Model file for the job. Use its own axes, mm. A direction names the side the tool comes from. Coordinates: 2 decimals unless noted, no trailing zeros. Order: outer loops, then holes, each group sorted by start corner. A loop starts at its lowest first (then second) coordinate and runs counter-clockwise, first axis right, second up. Notation, with made-up numbers: M -4,17 L 48,17 A32 cw 48,51 Z; hole C 11,44.5 d5. An arc over 180 degrees is marked long. Return JSON: item names as keys, results as strings.
```python
from build123d import *
from build123d.topology import SkipClean

# Parameters (mm, degrees)
SKETCH_1_R           = 19.5
SKETCH_1_R_2         = 18
EXTRUDE_1_DEPTH      = 20
SKETCH_3_R           = 27.5
EXTRUDE_2_DEPTH      = 3
EXTRUDE_START        = 2
SKETCH_25_R          = 21.75
SKETCH_25_R_2        = 19.5
EXTRUDE_12_DEPTH     = 2
EXTRUDE_START_2      = -1
SKETCH_26_R          = 21.75
SKETCH_26_R_2        = 19.5
EXTRUDE_13_DEPTH     = 2
EXTRUDE_START_3      = -3
EXTRUDE_14_DEPTH     = 3
SKETCH_28_W          = 21.458236434
SKETCH_28_H          = 3
SKETCH_28_W_2        = 3.541763566
EXTRUDE_17_DEPTH     = 1.5
EXTRUDE_START_4      = -53.5
EXTRUDE_25_DEPTH     = 53.5
CUT_EXTRUDE_START    = -52
CUT_EXTRUDE_15_DEPTH = 52
EXTRUDE_24_DEPTH     = 11
CUT_EXTRUDE_START_2  = -1.5
CUT_EXTRUDE_10_DEPTH = 1.5
SKETCH_34_W          = 10.2
SKETCH_34_H          = 6.5
SKETCH_34_W_2        = 8.2
SKETCH_34_H_2        = 4.5
EXTRUDE_22_DEPTH     = 5
SKETCH_37_W          = 8.2
SKETCH_37_H          = 4.5
CUT_EXTRUDE_9_DEPTH  = 5
EXTRUDE_26_DEPTH     = 8


with BuildPart() as part:
    # Sketch 1 → Extrude 1 (new body)
    with BuildSketch(Plane(origin=(0, 0, 0), x_dir=(1, 0, 0), z_dir=(0, 1, 0))):
        with Locations(Location((0, 0, 0), (0, 0, 270))):
            Circle(SKETCH_1_R)
        with Locations(Location((0, 0, 0), (0, 0, 270))):
            Circle(SKETCH_1_R_2, mode=Mode.SUBTRACT)
    extrude(amount=EXTRUDE_1_DEPTH)

    # Sketch 3 → Extrude 2 (add)
    with BuildSketch(Plane.XZ):
        with Locations(Location((0, 0, 0), (0, 0, 270))):
            Circle(SKETCH_3_R)
    extrude(amount=EXTRUDE_2_DEPTH)

    # Sketch 25 → Extrude 12 (add)
    with BuildSketch(Plane(origin=(0, 7, 0), x_dir=(-1, 0, 0), z_dir=(0, -1, 0)).offset(EXTRUDE_START)):
        with Locations(Location((0, 0, 0), (0, 0, 90))):
            Circle(SKETCH_25_R)
        with Locations(Location((0, 0, 0), (0, 0, 90))):
            Circle(SKETCH_25_R_2, mode=Mode.SUBTRACT)
    extrude(amount=-EXTRUDE_12_DEPTH)

    # Sketch 26 → Extrude 13 (add)
    with BuildSketch(Plane(origin=(0, 10.5, 0), x_dir=(-1, 0, 0), z_dir=(0, -1, 0)).offset(EXTRUDE_START_2)):
        with Locations(Location((0, 0, 0), (0, 0, 90))):
            Circle(SKETCH_26_R)
        with Locations(Location((0, 0, 0), (0, 0, 90))):
            Circle(SKETCH_26_R_2, mode=Mode.SUBTRACT)
    extrude(amount=-EXTRUDE_13_DEPTH)

    # Sketch 27 → Extrude 14 (add)
    with BuildSketch(Plane.XZ.offset(3).offset(EXTRUDE_START_3)):
        with BuildLine():
            Line((-12.5, 27.5), (-12.5, 24.494897428))
            ThreePointArc((-12.5, 24.494897428), (-6.428075946, 26.738171958), (0, 27.5))
            Line((0, 27.5), (-12.5, 27.5))
        make_face()
        with BuildLine():
            ThreePointArc((-8.958236434, -26), (-10.755478192, -25.309478241), (-12.5, -24.494897428))
            Line((-12.5, -24.494897428), (-12.5, -26))
            Line((-12.5, -26), (-8.958236434, -26))
        make_face()
        with BuildLine():
            ThreePointArc((0, 27.5), (6.428075946, 26.738171958), (12.5, 24.494897428))
            Line((12.5, 24.494897428), (12.5, 27.5))
            Line((12.5, 27.5), (0, 27.5))
        make_face()
        with BuildLine():
            Line((12.5, -26), (12.5, -24.494897428))
            ThreePointArc((12.5, -24.494897428), (10.755478192, -25.309478241), (8.958236434, -26))
            Line((8.958236434, -26), (12.5, -26))
        make_face()
    extrude(amount=EXTRUDE_14_DEPTH)

    # Sketch 28 → Extrude 17 (add)
    with BuildSketch(Plane(origin=(0, 0, -26), x_dir=(-1, 0, 0), z_dir=(0, 0, -1))):
        with BuildLine():
            Line((12.5, -38), (12.5, -3))
            Line((12.5, -3), (8.958236434, -3))
            Line((8.958236434, -3), (-12.5, -3))
            Line((-12.5, -3), (-12.5, -38))
            Line((-12.5, -38), (-8.6, -38))
            Line((-8.6, -38), (-8.6, -37.5))
            ThreePointArc((-8.6, -37.5), (-7.1, -36), (-5.6, -37.5))
            Line((-5.6, -37.5), (-5.6, -38))
            Line((-5.6, -38), (-4, -38))
            ThreePointArc((-4, -38), (0, -34), (4, -38))
            Line((4, -38), (5.6, -38))
            Line((5.6, -38), (5.6, -37.5))
            ThreePointArc((5.6, -37.5), (7.1, -36), (8.6, -37.5))
            Line((8.6, -37.5), (8.6, -38))
            Line((8.6, -38), (12.5, -38))
        make_face()
        with Locations((-1.770881783, -1.5)):
            Rectangle(SKETCH_28_W, SKETCH_28_H)
        with Locations((10.729118217, -1.5)):
            Rectangle(SKETCH_28_W_2, SKETCH_28_H)
        with BuildLine():
            ThreePointArc((-12.5, -38), (0, -50.5), (12.5, -38))
            Line((12.5, -38), (8.6, -38))
            Line((8.6, -38), (8.6, -38.5))
            ThreePointArc((8.6, -38.5), (7.1, -40), (5.6, -38.5))
            Line((5.6, -38.5), (5.6, -38))
            Line((5.6, -38), (4, -38))
            ThreePointArc((4, -38), (0, -42), (-4, -38))
            Line((-4, -38), (-5.6, -38))
            Line((-5.6, -38), (-5.6, -38.5))
            ThreePointArc((-5.6, -38.5), (-7.1, -40), (-8.6, -38.5))
            Line((-8.6, -38.5), (-8.6, -38))
            Line((-8.6, -38), (-12.5, -38))
        make_face()
    extrude(amount=EXTRUDE_17_DEPTH)

    # Sketch 28_25 → Extrude 25 (add)
    with BuildSketch(Plane(origin=(0, 0, -26), x_dir=(-1, 0, 0), z_dir=(0, 0, -1)).offset(EXTRUDE_START_4)):
        with BuildLine():
            Line((12.5, -38), (12.5, -3))
            Line((12.5, -3), (8.958236434, -3))
            Line((8.958236434, -3), (-12.5, -3))
            Line((-12.5, -3), (-12.5, -38))
            Line((-12.5, -38), (-8.6, -38))
            Line((-8.6, -38), (-8.6, -37.5))
            ThreePointArc((-8.6, -37.5), (-7.1, -36), (-5.6, -37.5))
            Line((-5.6, -37.5), (-5.6, -38))
            Line((-5.6, -38), (-4, -38))
            ThreePointArc((-4, -38), (0, -34), (4, -38))
            Line((4, -38), (5.6, -38))
            Line((5.6, -38), (5.6, -37.5))
            ThreePointArc((5.6, -37.5), (7.1, -36), (8.6, -37.5))
            Line((8.6, -37.5), (8.6, -38))
            Line((8.6, -38), (12.5, -38))
        make_face()
        with BuildLine():
            ThreePointArc((-12.5, -38), (0, -50.5), (12.5, -38))
            Line((12.5, -38), (8.6, -38))
            Line((8.6, -38), (8.6, -38.5))
            ThreePointArc((8.6, -38.5), (7.1, -40), (5.6, -38.5))
            Line((5.6, -38.5), (5.6, -38))
            Line((5.6, -38), (4, -38))
            ThreePointArc((4, -38), (0, -42), (-4, -38))
            Line((-4, -38), (-5.6, -38))
            Line((-5.6, -38), (-5.6, -38.5))
            ThreePointArc((-5.6, -38.5), (-7.1, -40), (-8.6, -38.5))
            Line((-8.6, -38.5), (-8.6, -38))
            Line((-8.6, -38), (-12.5, -38))
        make_face()
    extrude(amount=EXTRUDE_25_DEPTH)

    # Sketch 28_27 → Cut-Extrude 15 (cut)
    with BuildSketch(Plane(origin=(0, 0, -26), x_dir=(-1, 0, 0), z_dir=(0, 0, -1)).offset(CUT_EXTRUDE_START)):
        with BuildLine():
            ThreePointArc((-12.5, -38), (0, -50.5), (12.5, -38))
            Line((12.5, -38), (8.6, -38))
            Line((8.6, -38), (8.6, -38.5))
            ThreePointArc((8.6, -38.5), (7.1, -40), (5.6, -38.5))
            Line((5.6, -38.5), (5.6, -38))
            Line((5.6, -38), (4, -38))
            ThreePointArc((4, -38), (0, -42), (-4, -38))
            Line((-4, -38), (-5.6, -38))
            Line((-5.6, -38), (-5.6, -38.5))
            ThreePointArc((-5.6, -38.5), (-7.1, -40), (-8.6, -38.5))
            Line((-8.6, -38.5), (-8.6, -38))
            Line((-8.6, -38), (-12.5, -38))
        make_face()
        with BuildLine():
            Line((12.5, -38), (12.5, -3))
            Line((12.5, -3), (8.958236434, -3))
            Line((8.958236434, -3), (-12.5, -3))
            Line((-12.5, -3), (-12.5, -38))
            Line((-12.5, -38), (-8.6, -38))
            Line((-8.6, -38), (-8.6, -37.5))
            ThreePointArc((-8.6, -37.5), (-7.1, -36), (-5.6, -37.5))
            Line((-5.6, -37.5), (-5.6, -38))
            Line((-5.6, -38), (-4, -38))
            ThreePointArc((-4, -38), (0, -34), (4, -38))
            Line((4, -38), (5.6, -38))
            Line((5.6, -38), (5.6, -37.5))
            ThreePointArc((5.6, -37.5), (7.1, -36), (8.6, -37.5))
            Line((8.6, -37.5), (8.6, -38))
            Line((8.6, -38), (12.5, -38))
        make_face()
    extrude(amount=CUT_EXTRUDE_15_DEPTH, mode=Mode.SUBTRACT)

    # Sketch 38_4 → Extrude 24 (add)
    with BuildSketch(Plane(origin=(0, 0, -27.5), x_dir=(-1, 0, 0), z_dir=(0, 0, -1))):
        with BuildLine():
            Line((-1.3125, -15.961764662), (-1, -14.494677838))
            ThreePointArc((-1, -14.494677838), (-3.019933774, -6.069048379), (4.8, -9.8))
            ThreePointArc((4.8, -9.8), (3.730951621, -12.819933774), (1, -14.494677838))
            Line((1, -14.494677838), (1.3125, -15.961764662))
            ThreePointArc((1.3125, -15.961764662), (4.896874003, -13.763663079), (6.3, -9.8))
            ThreePointArc((6.3, -9.8), (-3.963663079, -4.903125997), (-1.3125, -15.961764662))
        make_face()
    extrude(amount=EXTRUDE_24_DEPTH)

    # Sketch 38 → Cut-Extrude 10 (cut)
    with SkipClean():  # the faces are left unmerged after this step: merging them gives an invalid solid
        with BuildSketch(Plane(origin=(0, 0, -27.5), x_dir=(-1, 0, 0), z_dir=(0, 0, -1)).offset(CUT_EXTRUDE_START_2)):
            with BuildLine():
                ThreePointArc((4.8, -9.8), (-3.019933774, -6.069048379), (-1, -14.494677838))
                ThreePointArc((-1, -14.494677838), (0, -14.6), (1, -14.494677838))
                ThreePointArc((1, -14.494677838), (3.730951621, -12.819933774), (4.8, -9.8))
            make_face()
        extrude(amount=CUT_EXTRUDE_10_DEPTH, mode=Mode.SUBTRACT)

    # Sketch 34 → Extrude 22 (add)
    with SkipClean():  # the faces are left unmerged after this step: merging them gives an invalid solid
        with BuildSketch(Plane(origin=(0, 0, 0), x_dir=(1, 0, 0), z_dir=(0, 1, 0))):
            with Locations((0, 9.75)):
                Rectangle(SKETCH_34_W, SKETCH_34_H)
            with Locations((0, 9.75)):
                Rectangle(SKETCH_34_W_2, SKETCH_34_H_2, mode=Mode.SUBTRACT)
        extrude(amount=EXTRUDE_22_DEPTH)

    # Sketch 37 → Cut-Extrude 9 (cut)
    with SkipClean():  # the faces are left unmerged after this step: merging them gives an invalid solid
        with BuildSketch(Plane(origin=(0, 0, 0), x_dir=(1, 0, 0), z_dir=(0, 1, 0))):
            with Locations((0, 9.75)):
                Rectangle(SKETCH_37_W, SKETCH_37_H)
        extrude(amount=-CUT_EXTRUDE_9_DEPTH, mode=Mode.SUBTRACT)

    # Sketch 38_12 → Extrude 26 (add)
    with SkipClean():  # the faces are left unmerged after this step: merging them gives an invalid solid
        with BuildSketch(Plane(origin=(0, 0, -27.5), x_dir=(-1, 0, 0), z_dir=(0, 0, -1))):
            with BuildLine():
                ThreePointArc((1, -14.494677838), (0, -14.6), (-1, -14.494677838))
                Line((-1, -14.494677838), (-1.3125, -15.961764662))
                ThreePointArc((-1.3125, -15.961764662), (0, -16.1), (1.3125, -15.961764662))
                Line((1.3125, -15.961764662), (1, -14.494677838))
            make_face()
            with BuildLine():
                Line((-1.3125, -15.961764662), (-1, -14.494677838))
                ThreePointArc((-1, -14.494677838), (-3.019933774, -6.069048379), (4.8, -9.8))
                ThreePointArc((4.8, -9.8), (3.730951621, -12.819933774), (1, -14.494677838))
                Line((1, -14.494677838), (1.3125, -15.961764662))
                ThreePointArc((1.3125, -15.961764662), (4.896874003, -13.763663079), (6.3, -9.8))
                ThreePointArc((6.3, -9.8), (-3.963663079, -4.903125997), (-1.3125, -15.961764662))
            make_face()
        extrude(amount=EXTRUDE_26_DEPTH)


solid = part.part
```
Item 1: Saw through at C-C (x = -15.5). Write the cut outline in (y, z), and give its area (3 significant figures).
Check result:
{"outline": "M -3,-22.72 L 0,-22.72 L 0,-11.83 L 5,-11.83 L 5,-15.26 L 7,-15.26 L 7,-11.83 L 11.5,-11.83 L 11.5,-15.26 L 13.5,-15.26 L 13.5,-11.83 L 20,-11.83 L 20,-9.15 L 0,-9.15 L 0,9.15 L 20,9.15 L 20,11.83 L 13.5,11.83 L 13.5,15.26 L 11.5,15.26 L 11.5,11.83 L 7,11.83 L 7,15.26 L 5,15.26 L 5,11.83 L 0,11.83 L 0,22.72 L -3,22.72 Z", "area": "271 mm2"}
Item 2: 3-axis set-ups, long thin cutter, end or side, ignore diameter. For faces 1 (the flat face through (-12.5, -19, 27)), 2 (the flat face through (-3.2, -6, -38.5)), 3 (the flat face through (-12.5, -19, -27)), 4 (the cylindrical face through (21.565, 5.986, 2.831)), 5 (the flat face through (-17.24, 20, 5.69)): which of +Z, -Z, +X, -X, +Y, -Y reach the whole face in a straight line?
Check result:
{"face 1": "+Z, -X, +Y, -Y", "face 2": "-Z, +X, -X, +Y, -Y", "face 3": "-Z, -X, +Y, -Y", "face 4": "+Y", "face 5": "+Z, -Z, +X, -X, +Y"}
Item 3: Saw through at B-B (z = 0). Write the cut outline in (x, y).
Check result:
{"outline": "M -27.5,-3 L 27.5,-3 L 27.5,0 L 19.5,0 L 19.5,5 L 21.75,5 L 21.75,7 L 19.5,7 L 19.5,11.5 L 21.75,11.5 L 21.75,13.5 L 19.5,13.5 L 19.5,20 L 18,20 L 18,0 L -18,0 L -18,20 L -19.5,20 L -19.5,13.5 L -21.75,13.5 L -21.75,11.5 L -19.5,11.5 L -19.5,7 L -21.75,7 L -21.75,5 L -19.5,5 L -19.5,0 L -27.5,0 Z"}
Item 4: Saw through at A-A (y = -23). Write the cut outline in (x, z).
Check result:
{"outline": "M -12.5,-27.5 L 12.5,-27.5 L 12.5,-26 L -12.5,-26 Z; M -12.5,26 L 12.5,26 L 12.5,27.5 L -12.5,27.5 Z"}
Item 5: Pull direction Y, two halves, no side cores. Call faces 6 (the cylindrical face through (19.334, 9.218, -2.539)), 7 (the flat face through (0, 2, -6.5)), 8 (the flat face through (18, 11.5, 8)), 9 (the cylindrical face through (0.275, -50.497, -26.74)): +Y half, -Y half, draft (parallel to the pull), parting line (faces both ways), or undercut.
Check result:
{"face 6": "undercut", "face 7": "draft", "face 8": "undercut", "face 9": "-Y half"}
Item 6: Drop flat-ended pins along their axis: pin 1 Ø13 at (x, y) = (0, -38) entering from +Z; pin 2 Ø4 at (y, z) = (-2, -13.5) entering from -X; pin 3 Ø6 at (x, y) = (19.5, 6) entering from -Z; pin 4 Ø0.5 at (y, z) = (-38, 26.5) entering from +X. Give the stop position or say it passes through.
Check result:
{"pin 1": "stops at z = 27.5", "pin 2": "stops at x = -24.98", "pin 3": "stops at z = -14.17", "pin 4": "stops at x = 12.5"}
Item 7: Wall check: line 1 (Y direction, x = 0, z = -27); line 2 (Y direction, x = 12.5, z = 15.5); line 3 (X direction, y = -38, z = -27). Give the ranges that are in metal, low to high.
Check result:
{"line 1": "y = -50.5 to -42, -34 to -14.6, -5 to 0", "line 2": "y = -3 to 0, 5 to 7, 11.5 to 13.5", "line 3": "x = -12.5 to -8.6, -5.6 to -4, 4 to 5.6, 8.6 to 12.5"}
